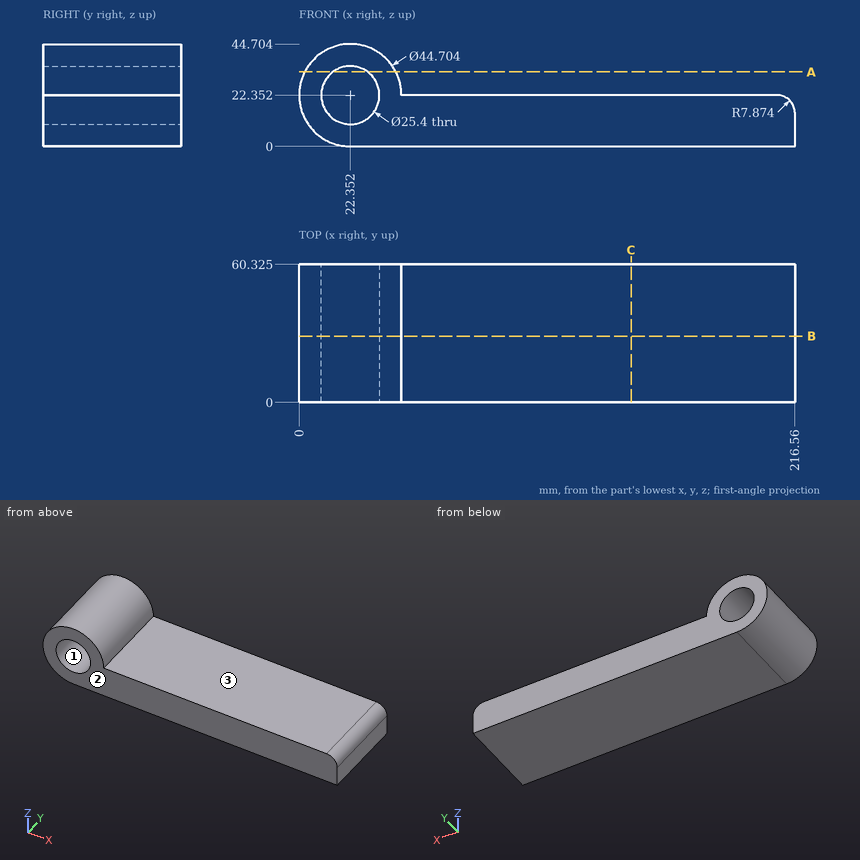
Input: dimensioned drawing with shaded views. Units: mm. Origin: part minimum x, y, z. Give positions to 0.01 mm unless a question says otherwise; leave off trailing zeros. Loops run counter-clockwise (first coordinate to the right, second up) from the corner with the lowest first, then second, coordinate; pieces in that order, holes last. Notation, with made-up numbers: (-35, 45.5) -> (-7, 45.5) arc R26 ccw to (-7, 76.5) -> close; hole circle Ø11 at (38, 29). An arc over 180 degrees is marked (long way). Use a Markdown table: item, result. Add a question column.
1) Section query A-A, the plane z = 32.5. Return the cut outline in (x, y) (1 decimal), then the cut area to 3 significant figures.
2) Line query: line 1 along Z through (x, y) = (127, 49.5); line 2 along X through (y, z) = (41.5, 28.5) (1 decimal); line 3 along X through (y, z) = (16, 32) (1 decimal). Output: solid intervals per line, ascending. Write a range as [from, to].
3) Section query C-C, the plane x = 145. Return the cut outline in (y, z) (1 decimal), then the cut area to 3 significant figures.
4) First-contact query: pin 1 (6 mm diameter, centred on y = 22, z = 7, fed in from -X); pin 2 (6 mm diameter, centred on y = 14.5, z = 30, fed in from -X). Flat tips, straight axial feed; report the tip coordinate or a pass-through.
5) Section query B-B, the plane y = 29. Return the cut outline in (x, z), then the cut area to 3 significant figures.
6) Pull-direction query (Z, two-part tool) for the marked faces 1, 2 and 3; classes: +Z half, -Z half, draft (parallel to the pull), parting line (faces both ways), or undercut.
Numbers:
| question | item | result |
|---|---|---|
| 1 | outline | (2.4, 0) -> (14.7, 0) -> (14.7, 60.3) -> (2.4, 60.3) -> close; (30, 0) -> (42.3, 0) -> (42.3, 60.3) -> (30, 60.3) -> close |
| 1 | area | 1,480 mm2 |
| 2 | line 1 | z = [0, 22.35] |
| 2 | line 2 | x = [0.9, 11.2], [33.5, 43.8] |
| 2 | line 3 | x = [2.2, 14.1], [30.6, 42.5] |
| 3 | outline | (0, 0) -> (60.3, 0) -> (60.3, 22.4) -> (0, 22.4) -> close |
| 3 | area | 1,350 mm2 |
| 4 | pin 1 | stops at x = 3.72 |
| 4 | pin 2 | stops at x = 0.49 |
| 5 | outline | (22.35, 0) -> (216.56, 0) -> (216.56, 14.48) arc R7.87 ccw to (208.69, 22.35) -> (44.7, 22.35) arc R22.35 ccw (long way) to start; hole circle Ø25.4 at (22.35, 22.35) |
| 5 | area | 5,000 mm2 |
| 6 | face 1 | undercut |
| 6 | face 2 | draft |
| 6 | face 3 | +Z half |
